Geometry check sheet. Reference: the model listing, model coordinates, mm. A direction names the side the tool comes from. Give positions to 0.01 mm unless a question says otherwise; leave off trailing zeros. Write each loop counter-clockwise with the first axis right and the second up, starting at its lowest first coordinate (ties: lowest second). Pieces come first, ordered by that corner, then holes. Notation, with made-up numbers: M 64,14 L 110,14 A20 cw 110,27 Z; hole C 24,-19 d11. An arc over 180 degrees is marked long. One line per item, written item: value. Start each with the question number.
1. Cross-section at B-B on y = 23. Record the cut outline in (x, z), then the cut area to 3 significant figures.
2. Tool access check on faces 1 (the face through (-1, 0, 0)), 2 (the face through (38, -33, 66.678)), 3 (the face through (-69.85, 0, 50)), 4 (the face through (-12.474, 32, 38)). Record the directions out of +Z, -Z, +X, -X, +Y, -Y that give a thin tool (end or side, any length) a straight path to the whole face; none if there is none.
3. Cross-section at A-A on x = -17.5. Record the cut outline in (y, z), then the cut area to 3 significant figures.
4. Scan lines: line 1 (X direction, y = -14, z = 41.5); line 2 (Z direction, x = -9.5, y = -17.5). Record each from-to range of solid material in increasing order.
5. Release check for a two-part mould opening along Y. For faces 5 (the face through (38, -30.067, 73)), 6 (the face through (-29.745, 32, 66)), 7 (the face through (1, -28.797, 50)) record: pulls with the +Y half, pulls with the -Y half, needs draft (parallel to the pull), parting line crosses it, or undercut.
6. Cross-section at C-C on x = 36. Record the cut outline in (y, z), then the cut area to 3 significant figures.
7. Cross-section at D-D on z = 36. Record the cut outline in (x, y).
from build123d import *

# Parameters (mm, degrees)
F0_W     = 152.4
F0_H     = 70.293026
F1_DEPTH = 12.7
F2_W     = 6.35
F2_H     = 57.593026
F3_DEPTH = 76.2
F4_W     = 25.4
F4_H     = 50.8
F4_H_2   = 12.7
F5_DEPTH = 6.35
F6_W     = 25.4
F6_H     = 12.7
F7_DEPTH = 5.08
F8_W     = 152.4
F8_H     = 70.293026
F9_DEPTH = 25.4


with BuildPart() as f1:
    # F0 (on Top) → F1 (new body)
    with BuildSketch(Plane.XY):
        Rectangle(F0_W, F0_H)
    extrude(amount=F1_DEPTH)

    # F2 (on face) → F3 (join)
    with BuildSketch(Plane.XY.offset(12.7)):
        Polygon((-70.562325, 35.146513), (-76.2, 35.146513), (-76.2, 28.796513), (-69.85, 28.796513), (69.85, 28.796513), (76.2, 28.796513), (76.2, 35.146513), (-63.181333, 35.146513), align=None)
        with Locations((-73.025, 0)):
            Rectangle(F2_W, F2_H)
        Polygon((-69.85, -28.796513), (-76.2, -28.796513), (-76.2, -35.146513), (76.2, -35.146513), (76.2, -28.796513), (69.85, -28.796513), align=None)
        with Locations((73.025, 0)):
            Rectangle(F2_W, F2_H)
    extrude(amount=F3_DEPTH)

    # F4 (on face) → F5 (cut, through all)
    with BuildSketch(Plane(origin=(0, 35.146513, 0), x_dir=(-1, 0, 0), z_dir=(0, 1, 0))):
        with Locations((-0.226117, 38.1)):
            Rectangle(F4_W, F4_H)
        with Locations((-44.232082, 66.113808)):
            Rectangle(F4_W, F4_H_2)
        with Locations((42.445415, 66.433654)):
            Rectangle(F4_W, F4_H_2)
    extrude(amount=-F5_DEPTH, mode=Mode.SUBTRACT)

    # F6 (on face) → F7 (cut)
    with BuildSketch(Plane.XZ.offset(35.146513)):
        with Locations((-51.077663, 73.014069)):
            Rectangle(F6_W, F6_H)
        with Locations((38.134995, 73.027868)):
            Rectangle(F6_W, F6_H)
    extrude(amount=-F7_DEPTH, mode=Mode.SUBTRACT)

    # F8 (on face) → F9 (join)
    with BuildSketch(Plane.XY.offset(88.9)):
        Rectangle(F8_W, F8_H)
    extrude(amount=F9_DEPTH)


solid = f1.part
Report:
1. outline: M -76.2,0 L 76.2,0 L 76.2,114.3 L -76.2,114.3 Z; hole M -69.85,12.7 L 69.85,12.7 L 69.85,88.9 L -69.85,88.9 Z
1. area: 6,770 mm^2
2. face 1: -Z, +X, -X, +Y, -Y
2. face 2: -Y
2. face 3: none
2. face 4: +Y
3. outline: M -35.15,0 L 35.15,0 L 35.15,114.3 L -35.15,114.3 Z; hole M -28.8,12.7 L 28.8,12.7 L 28.8,88.9 L -28.8,88.9 Z
3. area: 3,650 mm^2
4. line 1: x = -76.2 to -69.85, 69.85 to 76.2
4. line 2: z = 0 to 12.7, 88.9 to 114.3
5. face 5: pulls with the -Y half
5. face 6: needs draft
5. face 7: undercut
6. outline: M -35.15,0 L 35.15,0 L 35.15,59.76 L 28.8,59.76 L 28.8,12.7 L -28.8,12.7 L -28.8,88.9 L 28.8,88.9 L 28.8,72.46 L 35.15,72.46 L 35.15,114.3 L -35.15,114.3 L -35.15,79.38 L -30.07,79.38 L -30.07,66.68 L -35.15,66.68 Z
6. area: 3,500 mm^2
7. outline: M -76.2,-35.15 L 76.2,-35.15 L 76.2,35.15 L 12.93,35.15 L 12.93,28.8 L 69.85,28.8 L 69.85,-28.8 L -69.85,-28.8 L -69.85,28.8 L -12.47,28.8 L -12.47,35.15 L -76.2,35.15 Z
